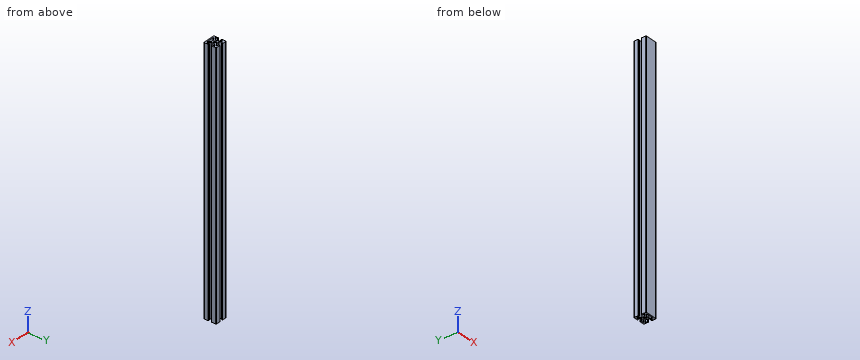
```python
from build123d import *

# Parameters (mm, degrees)
BOSS_EXTRUDE1_DEPTH = 260.35
FILLET2_R           = 0.254
FILLET1_R           = 1.27
SKETCH5_W           = 7.112
SKETCH5_H           = 2.54
BOSS_EXTRUDE2_DEPTH = 520.7


with BuildPart() as part:
    # Sketch3 → Boss-Extrude1 (new body, symmetric)
    with BuildSketch(Plane.XY):
        with BuildLine():
            Line((-12.7, 12.7), (-1.796051224, 1.796051224))
            ThreePointArc((-1.796051224, 1.796051224), (-0.972015918, 2.346654013), (0, 2.54))
            Line((0, 2.54), (0, 4.826))
            Line((0, 4.826), (-1.977846327, 4.826))
            ThreePointArc((-1.977846327, 4.826), (-2.949862246, 5.019345987), (-3.773897552, 5.569948776))
            Line((-3.773897552, 5.569948776), (-7.772528286, 9.56857951))
            ThreePointArc((-7.772528286, 9.56857951), (-7.847628361, 9.946133082), (-7.527553898, 10.16))
            Line((-7.527553898, 10.16), (-3.302, 10.16))
            Line((-3.302, 10.16), (-3.302, 12.7))
            Line((-3.302, 12.7), (-12.7, 12.7))
        make_face()
    extrude(amount=BOSS_EXTRUDE1_DEPTH, both=True)

    # Fillet2
    fillet2_edges = [part.edges().sort_by_distance(p)[0] for p in [
        (-3.302, 12.7, 0),
        (-3.302, 10.16, 0),
    ]]
    fillet(fillet2_edges, radius=FILLET2_R)

    # Mirror1: part across plane


with BuildPart() as part_1:
    add(part.part)
    add(part.part.mirror(Plane(origin=(0, 0, 260.35), x_dir=(0, 0, 1), z_dir=(0.707106781, 0.707106781, 0))))

    # Fillet1
    fillet1_edges = [part_1.edges().sort_by_distance(p)[0] for p in [
        (-12.7, 12.7, 0),
    ]]
    fillet(fillet1_edges, radius=FILLET1_R)

    # Mirror2: part across plane


with BuildPart() as part_2:
    add(part_1.part)
    add(part_1.part.mirror(Plane(origin=(0, 0, 260.35), x_dir=(0, 0, 1), z_dir=(0, 1, 0))))

    # Mirror5: part across plane


with BuildPart() as part_3:
    add(part_2.part)
    add(part_2.part.mirror(Plane(origin=(0, 0, 260.35), x_dir=(0, 0, 1), z_dir=(-1, 0, 0))))

    # Sketch5 → Boss-Extrude2 (add, through all)
    with BuildSketch(Plane.XY.offset(260.35)):
        with Locations((0, -11.43)):
            Rectangle(SKETCH5_W, SKETCH5_H)
    extrude(amount=-BOSS_EXTRUDE2_DEPTH)


solid = part_3.part
```
For this review, take the finished solid that the model builds, in its own axes (mm). Coordinates: 2 decimals unless noted, no trailing zeros. Answer in a Markdown table with one row per item. Add a question column.
Q1. We need section A-A, the plane z = 165. Count the separate pieces of the cut face and the enclosed holes in it, and give its area (3 significant figures).
Q2. For P1, Ø3, axis at x = -2, z = -99, coming from the +Y side; P2, Ø4.5, axis at x = 0.5, z = 122.5, coming from the +Y side; P3, Ø10, axis at y = 3.5, z = -120.5, coming from the +X side; P4, Ø2, axis at y = -1, z = 108, coming from the -X side, all flat-tipped, find the tip position at first contact; note any pin that passes through.
Q3. For probe 1 along Y at (x, z) = (-1.5, -44); probe 2 along X at (y, z) = (4.75, -145.5); probe 3 along Y at (x, z) = (-10.75, 232), list the stretches that pass through material, from the lowest coordinate up.
Answer list:
| question | item | result |
|---|---|---|
| 1 | separate pieces | 1 |
| 1 | enclosed holes | 2 |
| 1 | area | 332 mm2 |
| 2 | P1 | stops at y = 12.69 |
| 2 | P2 | stops at y = 4.95 |
| 2 | P3 | stops at x = 12.7 |
| 2 | P4 | stops at x = -4.83 |
| 3 | probe 1 | y = -12.7 to -10.16, -4.83 to -2.05, 2.05 to 4.83 |
| 3 | probe 2 | x = -12.7 to -10.16, -6.55 to 6.55, 10.16 to 12.7 |
| 3 | probe 3 | y = -12.7 to -3.3, 3.3 to 12.7 |
